Build history of the part. All positions in model axes, mm. Coordinates: 2 decimals unless noted, no trailing zeros. Loops run counter-clockwise (first coordinate to the right, second up) from the corner with the lowest first, then second, coordinate; pieces in that order, holes last. Notation, with made-up numbers: (-38.75, -12) -> (16.25, -12) arc R20 ccw to (16.25, -7) -> close; hole circle Ø2 at (-22.75, -4). An arc over 180 degrees is marked (long way). One line per item, written item: value. Start each with the question number.
```python
from build123d import *

# Parameters (mm, degrees)
SKETCH2_R           = 1.1
SKETCH2_W           = 14
SKETCH2_H           = 14
SKETCH2_W_2         = 13.999864793
SKETCH2_W_3         = 13.898443713
SKETCH2_W_4         = 14.000250013
SKETCH2_H_2         = 13.999122456
SKETCH2_H_3         = 13.99899745
SKETCH2_H_4         = 13.994084704
SKETCH2_W_5         = 16.66875
SKETCH2_H_5         = 16.66875
SKETCH2_H_6         = 40.48125
SKETCH2_W_6         = 8
SKETCH2_H_7         = 15
SKETCH2_W_7         = 15
SKETCH2_H_8         = 8
BOSS_EXTRUDE1_DEPTH = 1.5


with BuildPart() as part:
    # Sketch2 → Boss-Extrude1 (new body)
    with BuildSketch(Plane(origin=(0, 0, 0), x_dir=(0, 1, 0), z_dir=(0, 0, 1))):
        with BuildLine():
            Line((78.680047039, 95.509365468), (78.680047039, 69.315615468))
            Line((78.680047039, 69.315615468), (100.110297039, 69.315615468))
            Line((100.110297039, 69.315615468), (100.110297039, 95.563583947))
            Line((100.110297039, 95.563583947), (100.110297039, 97.890615468))
            Line((100.110297039, 97.890615468), (102.491547039, 97.890615468))
            Line((102.491547039, 97.890615468), (102.491547039, 95.509365468))
            Line((102.491547039, 95.509365468), (102.491547039, 66.884365468))
            Line((102.491547039, 66.884365468), (105.027080945, 64.348831562))
            ThreePointArc((105.027080945, 64.348831562), (106.110944702, 62.726714818), (106.491547039, 60.813297656))
            Line((106.491547039, 60.813297656), (106.491547039, 34.95543328))
            ThreePointArc((106.491547039, 34.95543328), (106.110944702, 33.042016118), (105.027080945, 31.419899374))
            Line((105.027080945, 31.419899374), (102.491547039, 28.884365468))
            Line((102.491547039, 28.884365468), (102.491547039, 0.259365468))
            Line((102.491547039, 0.259365468), (102.491547039, -2.121884532))
            Line((102.491547039, -2.121884532), (69.102852155, -2.121884532))
            Line((69.102852155, -2.121884532), (66.567318249, -4.657418438))
            ThreePointArc((66.567318249, -4.657418438), (64.945201505, -5.741282195), (63.031784343, -6.121884532))
            Line((63.031784343, -6.121884532), (37.173919967, -6.121884532))
            ThreePointArc((37.173919967, -6.121884532), (35.260502805, -5.741282195), (33.638386061, -4.657418438))
            Line((33.638386061, -4.657418438), (31.102852155, -2.121884532))
            Line((31.102852155, -2.121884532), (-2.285842729, -2.121884532))
            Line((-2.285842729, -2.121884532), (-2.285842729, 28.884365468))
            Line((-2.285842729, 28.884365468), (-4.821376635, 31.419899374))
            ThreePointArc((-4.821376635, 31.419899374), (-5.905240392, 33.042016118), (-6.285842729, 34.95543328))
            Line((-6.285842729, 34.95543328), (-6.285842729, 60.813297656))
            ThreePointArc((-6.285842729, 60.813297656), (-5.905240392, 62.726714818), (-4.821376635, 64.348831562))
            Line((-4.821376635, 64.348831562), (-2.285842729, 66.884365468))
            Line((-2.285842729, 66.884365468), (-2.285842729, 97.890615468))
            Line((-2.285842729, 97.890615468), (31.102852155, 97.890615468))
            Line((31.102852155, 97.890615468), (33.638386061, 100.426149374))
            ThreePointArc((33.638386061, 100.426149374), (35.260502805, 101.510013131), (37.173919967, 101.890615468))
            Line((37.173919967, 101.890615468), (63.031784343, 101.890615468))
            ThreePointArc((63.031784343, 101.890615468), (64.945201505, 101.510013131), (66.567318249, 100.426149374))
            Line((66.567318249, 100.426149374), (69.102852155, 97.890615468))
            Line((69.102852155, 97.890615468), (78.680047039, 97.890615468))
            Line((78.680047039, 97.890615468), (78.680047039, 95.509365468))
        make_face()
        with Locations(Location((19.145407271, 76.459365468, 0), (0, 0, 270))):
            Circle(SKETCH2_R, mode=Mode.SUBTRACT)
        with Locations(Location((19.145407271, 19.309365468, 0), (0, 0, 270))):
            Circle(SKETCH2_R, mode=Mode.SUBTRACT)
        with Locations(Location((76.298797039, 38.359365468, 0), (0, 0, 270))):
            Circle(SKETCH2_R, mode=Mode.SUBTRACT)
        with Locations((19.145407271, 9.783779189)):
            Rectangle(SKETCH2_W, SKETCH2_H, mode=Mode.SUBTRACT)
        with Locations((47.721668484, 9.783779189)):
            Rectangle(SKETCH2_W_2, SKETCH2_H, mode=Mode.SUBTRACT)
        with Locations((66.721910491, 19.309365468)):
            Rectangle(SKETCH2_W_3, SKETCH2_H, mode=Mode.SUBTRACT)
        with Locations((9.619905995, 28.834302965)):
            Rectangle(SKETCH2_W_4, SKETCH2_H_2, mode=Mode.SUBTRACT)
        with Locations((28.67078354, 28.834302965)):
            Rectangle(SKETCH2_W, SKETCH2_H_2, mode=Mode.SUBTRACT)
        with Locations((47.721668484, 28.834302965)):
            Rectangle(SKETCH2_W_2, SKETCH2_H_2, mode=Mode.SUBTRACT)
        with Locations((9.619905995, 47.884365468)):
            Rectangle(SKETCH2_W_4, SKETCH2_H_3, mode=Mode.SUBTRACT)
        with Locations((28.67078354, 47.884365468)):
            Rectangle(SKETCH2_W, SKETCH2_H_3, mode=Mode.SUBTRACT)
        with Locations((47.721668484, 47.884365468)):
            Rectangle(SKETCH2_W_2, SKETCH2_H_3, mode=Mode.SUBTRACT)
        with Locations((66.721910491, 57.409365468)):
            Rectangle(SKETCH2_W_3, SKETCH2_H, mode=Mode.SUBTRACT)
        with Locations((9.619905995, 66.933889194)):
            Rectangle(SKETCH2_W_4, SKETCH2_H_4, mode=Mode.SUBTRACT)
        with Locations((28.67078354, 66.933889194)):
            Rectangle(SKETCH2_W, SKETCH2_H_4, mode=Mode.SUBTRACT)
        with Locations((47.721668484, 66.933889194)):
            Rectangle(SKETCH2_W_2, SKETCH2_H_4, mode=Mode.SUBTRACT)
        with Locations((9.619905995, 85.98779939)):
            Rectangle(SKETCH2_W_4, SKETCH2_H, mode=Mode.SUBTRACT)
        with Locations((28.67078354, 85.98779939)):
            Rectangle(SKETCH2_W, SKETCH2_H, mode=Mode.SUBTRACT)
        with Locations((47.721668484, 85.98779939)):
            Rectangle(SKETCH2_W_2, SKETCH2_H, mode=Mode.SUBTRACT)
        with Locations((66.721910491, 85.98779939)):
            Rectangle(SKETCH2_W_3, SKETCH2_H, mode=Mode.SUBTRACT)
        with Locations((89.395672039, 58.599990468)):
            Rectangle(SKETCH2_W_5, SKETCH2_H_5, mode=Mode.SUBTRACT)
        with Locations((89.395672039, 25.262490468)):
            Rectangle(SKETCH2_W_5, SKETCH2_H_6, mode=Mode.SUBTRACT)
        with Locations((31.045407271, 9.283779189)):
            Rectangle(SKETCH2_W_6, SKETCH2_H_7, mode=Mode.SUBTRACT)
        with Locations((7.245407271, 9.283779189)):
            Rectangle(SKETCH2_W_6, SKETCH2_H_7, mode=Mode.SUBTRACT)
        with Locations((67.272688635, 31.209365468)):
            Rectangle(SKETCH2_W_7, SKETCH2_H_8, mode=Mode.SUBTRACT)
        with Locations((67.272688635, 7.409365468)):
            Rectangle(SKETCH2_W_7, SKETCH2_H_8, mode=Mode.SUBTRACT)
        with Locations((67.272688635, 45.509365468)):
            Rectangle(SKETCH2_W_7, SKETCH2_H_8, mode=Mode.SUBTRACT)
        with Locations((67.272688635, 69.309365468)):
            Rectangle(SKETCH2_W_7, SKETCH2_H_8, mode=Mode.SUBTRACT)
    extrude(amount=BOSS_EXTRUDE1_DEPTH)


solid = part.part
```
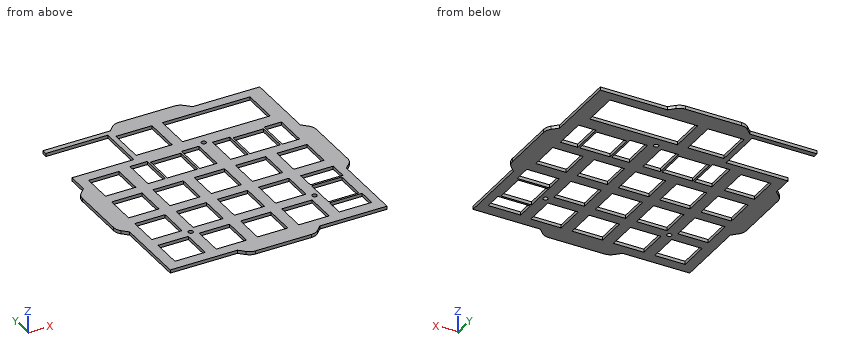
Item 1: Band-saw the part on C-C, the plane x = -53.5. List the corners of the cut face in (y, z), and give its area (3 significant figures).
Item 2: Band-saw the part on A-A, the plane y = 95.5. List the corners of the cut face in (x, z), and give its area (3 significant figures).
Item 3: Drop flat-ended pins along their axis: pin 1 Ø3 at (x, y) = (-42, 13) entering from -Z; pin 2 Ø0.8 at (y, z) = (8, 1) entering from -X; pin 3 Ø0.8 at (x, z) = (-13, 1) entering from -Y. Give the stop position or say it passes through.
Item 4: Probe probe 1 along Y at (x, z) = (-85.5, 0.65); probe 2 along X at (y, z) = (50.5, 0.15); probe 3 along Y at (x, z) = (-19.5, 1.45). List the from-to ranges inside material, lowest first.
Item 5: Band-saw the part on D-D, the plane z = 0.6. Count the separate pieces of the cut face and the enclosed holes in it, and give its area (3 significant figures).
Item 6: Band-saw the part on B-B, the plane y = 49.5. List the corners of the cut face in (x, z).
Worked out:
1. outline: (-6.29, 0) -> (2.62, 0) -> (2.62, 1.5) -> (-6.29, 1.5) -> close; (16.62, 0) -> (21.67, 0) -> (21.67, 1.5) -> (16.62, 1.5) -> close; (35.67, 0) -> (40.72, 0) -> (40.72, 1.5) -> (35.67, 1.5) -> close; (54.72, 0) -> (59.77, 0) -> (59.77, 1.5) -> (54.72, 1.5) -> close; (73.67, 0) -> (81.06, 0) -> (81.06, 1.5) -> (73.67, 1.5) -> close; (97.73, 0) -> (106.49, 0) -> (106.49, 1.5) -> (97.73, 1.5) -> close
1. area: 60.3 mm²
2. outline: (-69.32, 0) -> (-66.93, 0) -> (-66.93, 1.5) -> (-69.32, 1.5) -> close; (-50.27, 0) -> (-45.5, 0) -> (-45.5, 1.5) -> (-50.27, 1.5) -> close; (-5.02, 0) -> (2.12, 0) -> (2.12, 1.5) -> (-5.02, 1.5) -> close
2. area: 21.4 mm²
3. pin 1: stops at z = 0
3. pin 2: stops at x = -97.89
3. pin 3: stops at y = -2.29
4. probe 1: y = -2.29 to 2.62, 16.62 to 21.67, 35.67 to 40.72, 54.72 to 59.77, 73.67 to 78.68, 100.11 to 102.49
4. probe 2: x = -101.89 to -92.99, -78.99 to -73.93, -59.94 to -54.88, -40.88 to -35.83, -21.83 to -16.78, -2.78 to 6.12
4. probe 3: y = -2.29 to 18.06, 20.23 to 59.77, 73.67 to 81.06, 97.73 to 102.49
5. separate pieces: 1
5. enclosed holes: 28
5. area: 5,390 mm²
6. outline: (-101.89, 0) -> (-92.99, 0) -> (-92.99, 1.5) -> (-101.89, 1.5) -> close; (-78.99, 0) -> (-73.93, 0) -> (-73.93, 1.5) -> (-78.99, 1.5) -> close; (-59.94, 0) -> (-54.88, 0) -> (-54.88, 1.5) -> (-59.94, 1.5) -> close; (-40.88, 0) -> (-35.83, 0) -> (-35.83, 1.5) -> (-40.88, 1.5) -> close; (-21.83, 0) -> (-16.78, 0) -> (-16.78, 1.5) -> (-21.83, 1.5) -> close; (-2.78, 0) -> (6.12, 0) -> (6.12, 1.5) -> (-2.78, 1.5) -> close
